from build123d import *

# Parameters (mm, degrees)
EXTRUDE1_DEPTH = 5
EXTRUDE2_REACH = 169.33
SKETCH2_R      = 6


with BuildPart() as part:
    # Sketch1 → Extrude1 (new body)
    with BuildSketch(Plane(origin=(0, 0, 0), x_dir=(1, 0, 0), z_dir=(0, 1, 0))):
        with BuildLine():
            Line((-107.892566896, 91.758035695), (0, 23.652571955))
            Line((0, 23.652571955), (107.892566896, 91.758035695))
            ThreePointArc((107.892566896, 91.758035695), (135.320402304, 84.500183199), (127.892548484, 57.117897581))
            Line((127.892548484, 57.117897581), (19.999981588, -10.987566159))
            Line((19.999981588, -10.987566159), (19.999981588, -74.472862077))
            ThreePointArc((19.999981588, -74.472862077), (0, -94.5), (-19.999981588, -74.472862077))
            Line((-19.999981588, -74.472862077), (-19.999981588, -10.987566159))
            Line((-19.999981588, -10.987566159), (-127.892548484, 57.117897581))
            ThreePointArc((-127.892548484, 57.117897581), (-135.320402304, 84.500183199), (-107.892566896, 91.758035695))
        make_face()
    extrude(amount=EXTRUDE1_DEPTH)

    # Sketch2 → Extrude2 (cut, up to next)
    with BuildSketch(Plane(origin=(0, 5, 0), x_dir=(-1, 0, 0), z_dir=(0, 1, 0)), mode=Mode.PRIVATE) as extrude2_sk1:
        with Locations(Location((118, -74.5, 0), (0, 0, 90))):
            Circle(SKETCH2_R)
    extrude2_tool1 = extrude(extrude2_sk1.sketch, amount=-EXTRUDE2_REACH, mode=Mode.PRIVATE) & part.part
    # Sketch2 → Extrude2 (cut, up to next)
    with BuildSketch(Plane(origin=(0, 5, 0), x_dir=(-1, 0, 0), z_dir=(0, 1, 0)), mode=Mode.PRIVATE) as extrude2_sk2:
        with Locations(Location((-118, -74.5, 0), (0, 0, 90))):
            Circle(SKETCH2_R)
    extrude2_tool2 = extrude(extrude2_sk2.sketch, amount=-EXTRUDE2_REACH, mode=Mode.PRIVATE) & part.part
    # Sketch2 → Extrude2 (cut, up to next)
    with BuildSketch(Plane(origin=(0, 5, 0), x_dir=(-1, 0, 0), z_dir=(0, 1, 0)), mode=Mode.PRIVATE) as extrude2_sk3:
        with Locations(Location((0, 74.5, 0), (0, 0, 90))):
            Circle(SKETCH2_R)
    extrude2_tool3 = extrude(extrude2_sk3.sketch, amount=-EXTRUDE2_REACH, mode=Mode.PRIVATE) & part.part
    add(extrude2_tool1.solids().sort_by_distance((-118, 5, -74.5))[0], mode=Mode.SUBTRACT)
    add(extrude2_tool2.solids().sort_by_distance((118, 5, -74.5))[0], mode=Mode.SUBTRACT)
    add(extrude2_tool3.solids().sort_by_distance((0, 5, 74.5))[0], mode=Mode.SUBTRACT)


solid = part.part
Design review of the part built by this model. Coordinates are the model's own, in mm. A direction names the side the tool comes from. Round coordinates to 2 decimals unless told otherwise and drop trailing zeros. Write each loop counter-clockwise with the first axis right and the second up, starting at its lowest first coordinate (ties: lowest second). Pieces come first, ordered by that corner, then holes.
Item 1: Wall thickness on L1, parallel to X at y = 3.85, z = -74.5; L2, parallel to X at y = 2.9, z = 74.5; L3, parallel to X at y = 3.4, z = 33.5: over which ranges is each line inside the solid? List them lowest first.
Item 2: Consider section D-D on z = 62. Give the boundary of the cut face in (x, y).
Item 3: For faces 1 (the flat face through (-73.19, 2.46, -22.59)), 2 (the flat face through (-54.7, 2.46, -58.18)), list the 3-axis set-ups (+Z, -Z, +X, -X, +Y, -Y) from which the entire face can be reached by the end or side of a thin tool; tool diameter is ignored.
Item 4: Consider section C-C on z = -76.5. Give the boundary of the cut face in (x, y).
Item 5: Consider section A-A on y = 1.25. Give the boundary of the cut face in (x, z).
Item 6: For pin 1 Ø7 at (x, z) = (118, -74.5) entering from +Y; pin 2 Ø1.5 at (y, z) = (4.5, 26.5) entering from +X; pin 3 Ø2 at (x, y) = (27, 2.5) entering from -Z; pin 4 Ø3 at (x, y) = (28, 1) entering from -Z, all flat-tipped, find the tip position at first contact; note any pin that passes through.
Item 7: Consider section B-B on x = -118. Give the boundary of the cut face in (y, z).
Item 8: Draft analysis for pull direction Z (two halves, no side actions). For faces 3 (the flat face through (74.7, 2.46, -23.54)), 4 (the flat face through (11, 0, -21)), 5 (the cylindrical face through (-113.94, 2.54, -78.92)), 6 (the cylindrical face through (0.264, 2.535, 68.506)), state which applies: released by +Z, released by -Z, zero draft, split by the parting line, or undercut.
Check values:
1. L1: x = -138 to -124, -112 to -80.55, 80.55 to 112, 124 to 138
1. L2: x = -20 to -6, 6 to 20
1. L3: x = -20 to 20
2. outline: (-20, 0) - (20, 0) - (20, 5) - (-20, 5) - close
3. face 1: +Z, -X, +Y, -Y
3. face 2: -Z, +Y, -Y
4. outline: (-137.9, 0) - (-123.66, 0) - (-123.66, 5) - (-137.9, 5) - close; (-112.34, 0) - (-83.72, 0) - (-83.72, 5) - (-112.34, 5) - close; (83.72, 0) - (112.34, 0) - (112.34, 5) - (83.72, 5) - close; (123.66, 0) - (137.9, 0) - (137.9, 5) - (123.66, 5) - close
5. outline: (-127.89, -57.12) arc R20 ccw (long way) to (-107.89, -91.76) - (0, -23.65) - (107.89, -91.76) arc R20 ccw (long way) to (127.89, -57.12) - (20, 10.99) - (20, 74.47) arc R20 ccw to (-20, 74.47) - (-20, 10.99) - close; hole circle Ø12 at (-118, -74.5); hole circle Ø12 at (0, 74.5); hole circle Ø12 at (118, -74.5)
6. pin 1: passes through
6. pin 2: stops at x = 20
6. pin 3: stops at z = -41.33
6. pin 4: stops at z = -42.27
7. outline: (0, -94.5) - (5, -94.5) - (5, -80.5) - (0, -80.5) - close; (0, -68.5) - (5, -68.5) - (5, -50.87) - (0, -50.87) - close
8. face 3: released by +Z
8. face 4: zero draft
8. face 5: undercut
8. face 6: undercut
